Design review of the part shown in the three views and the two pictorial views. Dimensions are in mm from the part's minimum x, y and z. A direction names the side the tool comes from. Round coordinates to 2 decimals unless told otherwise and drop trailing zeros. Loops run counter-clockwise (first coordinate to the right, second up) from the corner with the lowest first, then second, coordinate; pieces in that order, holes last. Notation, with made-up numbers: M 79.5,-1.75 L 132.5,-1.75 A22 cw 132.5,31.25 Z; hole C -30,-14.75 d11. An arc over 180 degrees is marked long. One line per question, with ' | ' between items. Start each with the question number.
1) We need section C-C (y = 96.5). Give the boundary of the cut face in (x, z) (3 decimals).
2) For probe 1 along Y at (x, z) = (7.25, 91); probe 2 along X at (y, z) = (80, 23.5) (3 decimals), list the stretches that pass through material, from the lowest coordinate up. Write a range as from..to.
3) For the marked faces 1 and 2, list the 3-axis set-ups (+Z, -Z, +X, -X, +Y, -Y) from which the entire face can be reached by the end or side of a thin tool; tool diameter is ignored.
4) We need section A-A (x = 5.25). Give the boundary of the cut face in (y, z), and give its area (3 significant figures).
5) For pin 1 Ø8 at (y, z) = (93.5, 74.5) entering from -X (3 decimals), flat-tipped, find the tip position at first contact; note if it passes through.
6) Mouldability with a two-part tool opening along Y and no side actions: class the marked faces 3, 4 and 5 as pulls with the +Y half, pulls with the -Y half, needs draft (parallel to the pull), parting line crosses it, or undercut.
7) We need section B-B (z = 49). Give the boundary of the cut face in (x, y) (3 decimals).
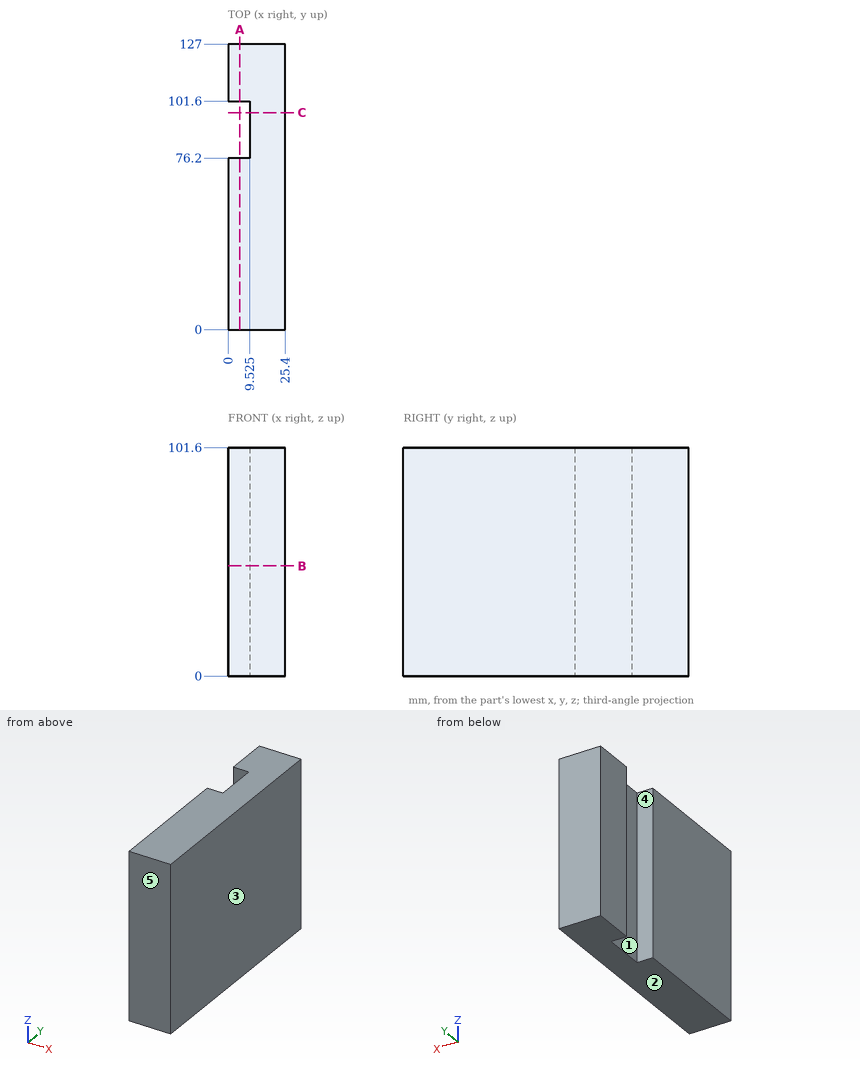
Answers below:
1) outline: M 9.525,0 L 25.4,0 L 25.4,101.6 L 9.525,101.6 Z
2) probe 1: 0..76.2, 101.6..127 | probe 2: 9.525..25.4
3) face 1: +Z, -Z, -X | face 2: -Z, +X, -X, +Y, -Y
4) outline: M 0,0 L 76.2,0 L 76.2,101.6 L 0,101.6 Z; M 101.6,0 L 127,0 L 127,101.6 L 101.6,101.6 Z | area: 10,300 mm^2
5) pin 1: x = 9.525
6) face 3: needs draft | face 4: undercut | face 5: pulls with the -Y half
7) outline: M 0,0 L 25.4,0 L 25.4,127 L 0,127 L 0,101.6 L 9.525,101.6 L 9.525,76.2 L 0,76.2 Z
